```python
from build123d import *

# Parameters (mm, degrees)
SKETCH1_R           = 20
SKETCH1_R_2         = 10
BOSS_EXTRUDE2_DEPTH = 15
FILLET1_R           = 1
FILLET2_R           = 1
FILLET3_R           = 1


with BuildPart() as part:
    # Sketch1 → Boss-Extrude2 (new body)
    with BuildSketch(Plane(origin=(0, 0, 0), x_dir=(1, 0, 0), z_dir=(0, 1, 0))):
        Circle(SKETCH1_R)
        Circle(SKETCH1_R_2, mode=Mode.SUBTRACT)
    extrude(amount=BOSS_EXTRUDE2_DEPTH)

    # Fillet1
    fillet1_edges = [part.edges().sort_by_distance(p)[0] for p in [
        (-20, 15, 0),
    ]]
    fillet(fillet1_edges, radius=FILLET1_R)

    # Fillet2
    fillet2_edges = [part.edges().sort_by_distance(p)[0] for p in [
        (-10, 15, 0),
    ]]
    fillet(fillet2_edges, radius=FILLET2_R)

    # Fillet3
    fillet3_edges = [part.edges().sort_by_distance(p)[0] for p in [
        (-20, 0, 0),
        (-10, 0, 0),
    ]]
    fillet(fillet3_edges, radius=FILLET3_R)


solid = part.part
```
CAD build for the part. Positions are in the model's coordinates, mm. Round coordinates to 2 decimals unless told otherwise and drop trailing zeros. Loops run counter-clockwise (first coordinate to the right, second up) from the corner with the lowest first, then second, coordinate; pieces in that order, holes last. Notation, with made-up numbers: M 55,-33.5 L 112,-33.5 A14 ccw 112,-14.5 Z; hole C 51.25,-17 d11. An arc over 180 degrees is marked long. Return JSON: item names as keys, results as strings. Group by question number.
(1) Wall check: probe 1 along X at (y, z) = (5.75, 0); probe 2 along X at (y, z) = (5.5, 7) (3 decimals). Give the ranges that are in metal, low to high. Write a range as [from, to].
(2) Drop flat-ended pins along their axis: P1, Ø6, axis at x = -10.5, z = 2.5, coming from the +Y side; P2, Ø6, axis at x = 4.5, y = 6, coming from the -Z side; P3, Ø8, axis at x = 14.5, y = 13, coming from the -Z side; P4, Ø6, axis at x = -14.5, y = 4.5, coming from the +Z side. Give the stop position or say it passes through.
(3) Saw through at B-B, the plane x = 0. List the corners of the cut face in (y, z), and give its area (3 significant figures).
(4) Saw through at C-C, the plane y = 9. List the corners of the cut face in (x, z).
(5) Saw through at A-A, the plane z = 0. List the corners of the cut face in (x, y).
(6) Mould opens along X. For faces 1 (the cylindrical face through (-2.17, 7.41, 9.76)), 2 (the flat face through (8, 15, 8)), 3 (the cylindrical face through (-4.336, 7.409, 19.524)) say: +X half, -X half, draft (parallel to the pull), parting line (faces both ways), or undercut.
Answer list:
{
 "1": {"probe 1": "[-20, -10], [10, 20]", "probe 2": "[-18.735, -7.141], [7.141, 18.735]"},
 "2": {"P1": "y = 15", "P2": "z = -19.94", "P3": "z = -17.02", "P4": "z = 16.36"},
 "3": {"outline": "M 0,-19 A1 ccw 1,-20 L 14,-20 A1 ccw 15,-19 L 15,-11 A1 ccw 14,-10 L 1,-10 A1 ccw 0,-11 Z; M 0,11 A1 ccw 1,10 L 14,10 A1 ccw 15,11 L 15,19 A1 ccw 14,20 L 1,20 A1 ccw 0,19 Z", "area": "298 mm2"},
 "4": {"outline": "C 0,0 d40; hole C 0,0 d20"},
 "5": {"outline": "M -20,1 A1 ccw -19,0 L -11,0 A1 ccw -10,1 L -10,14 A1 ccw -11,15 L -19,15 A1 ccw -20,14 Z; M 10,1 A1 ccw 11,0 L 19,0 A1 ccw 20,1 L 20,14 A1 ccw 19,15 L 11,15 A1 ccw 10,14 Z"},
 "6": {"face 1": "undercut", "face 2": "draft", "face 3": "parting line"}
}
